```python
from build123d import *

# Parameters (mm, degrees)
SKETCH_1_W          = 70
SKETCH_1_H          = 40
EXTRUDE_1_DEPTH     = 5
CUT_EXTRUDE_1_DEPTH = 5
FILLET_1_R          = 2
SKETCH_3_W          = 23.333333333
SKETCH_3_H          = 4.8
EXTRUDE_2_DEPTH     = 5
FILLET_2_R          = 1
SKETCH_4_R          = 1.1
CUT_EXTRUDE_2_DEPTH = 5
HOLE_WIZARD_M3_1_D  = 3.4


with BuildPart() as part:
    # 草图1 → 凸台-拉伸1 (new body)
    with BuildSketch(Plane(origin=(0, 0, 0), x_dir=(0, 0, -1), z_dir=(1, 0, 0))):
        with Locations((35, 20)):
            Rectangle(SKETCH_1_W, SKETCH_1_H)
    extrude(amount=EXTRUDE_1_DEPTH)

    # 草图2 → 切除-拉伸1 (cut)
    with BuildSketch(Plane(origin=(5, 0, 0), x_dir=(0, 0, -1), z_dir=(1, 0, 0))):
        Polygon((8, 8), (24, 8), (8, 32), align=None)
        Polygon((31, 32), (31, 8), (15, 32), align=None)
        Polygon((39, 32), (39, 8), (55, 32), align=None)
        Polygon((62, 8), (62, 32), (46, 8), align=None)
    extrude(amount=-CUT_EXTRUDE_1_DEPTH, mode=Mode.SUBTRACT)

    # 圆角1
    fillet_1_edges = [part.edges().sort_by_distance(p)[0] for p in [
        (2.5, 32, -31),
        (2.5, 8, -31),
        (2.5, 32, -15),
        (2.5, 8, -39),
        (2.5, 32, -39),
        (2.5, 32, -55),
        (2.5, 32, -62),
        (2.5, 8, -62),
        (2.5, 8, -46),
        (2.5, 8, -8),
        (2.5, 32, -8),
        (2.5, 8, -24),
    ]]
    fillet(fillet_1_edges, radius=FILLET_1_R)

    # 草图3 → 凸台-拉伸2 (add)
    with BuildSketch(Plane(origin=(5, 0, 0), x_dir=(0, 0, -1), z_dir=(1, 0, 0))):
        with Locations((11.666666667, 42.4)):
            Rectangle(SKETCH_3_W, SKETCH_3_H)
        with Locations((58.333333334, 42.4)):
            Rectangle(SKETCH_3_W, SKETCH_3_H)
        with Locations((58.333333334, -2.4)):
            Rectangle(SKETCH_3_W, SKETCH_3_H)
        with Locations((11.666666667, -2.4)):
            Rectangle(SKETCH_3_W, SKETCH_3_H)
    extrude(amount=-EXTRUDE_2_DEPTH)

    # 圆角2
    fillet_2_edges = [part.edges().sort_by_distance(p)[0] for p in [
        (2.5, 44.8, 0),
        (2.5, 44.8, -23.333333333),
        (2.5, 44.8, -70),
        (2.5, 44.8, -46.666666667),
        (2.5, -4.8, -23.333333333),
        (2.5, -4.8, 0),
        (2.5, -4.8, -70),
        (2.5, -4.8, -46.666666667),
    ]]
    fillet(fillet_2_edges, radius=FILLET_2_R)

    # 草图4 → 切除-拉伸2 (cut)
    with BuildSketch(Plane(origin=(5, 0, 0), x_dir=(0, 0, -1), z_dir=(1, 0, 0))):
        with Locations((23.333333333, 40)):
            Circle(SKETCH_4_R)
        with Locations((46.666666667, 40)):
            Circle(SKETCH_4_R)
        with Locations((46.666666667, 0)):
            Circle(SKETCH_4_R)
        with Locations((23.333333333, 0)):
            Circle(SKETCH_4_R)
    extrude(amount=-CUT_EXTRUDE_2_DEPTH, mode=Mode.SUBTRACT)

    # M3 间隙孔1 (through all)
    with Locations(Plane(origin=(5, 0, 0), x_dir=(0, 0, -1), z_dir=(1, 0, 0))):
        with Locations((57.5, 37), (47.5, 37), (57.5, 3), (47.5, 3), (22.5, 3), (12.5, 3), (22.5, 37), (12.5, 37)):
            Hole(HOLE_WIZARD_M3_1_D / 2)


solid = part.part
```
Here's how the part is built. I have some questions about the finished solid (model axes, mm). Coordinates: 2 decimals unless noted, no trailing zeros. Order: outer loops, then holes, each group sorted by start corner. A loop starts at its lowest first (then second) coordinate and runs counter-clockwise, first axis right, second up. Notation, with made-up numbers: (24.5, -37.5) -> (73.5, -37.5) arc R35 cw to (73.5, -4.5) -> close; hole circle Ø5 at (62.25, -24.75). An arc over 180 degrees is marked (long way). Return JSON: item names as keys, results as strings.
1) If we section it at B-B on z = -15: List the corners of the cut face in (x, y) for me.
Conclusion:
{"outline": "(0, -4.8) -> (5, -4.8) -> (5, 8) -> (0, 8) -> close; (0, 21.5) -> (5, 21.5) -> (5, 44.8) -> (0, 44.8) -> close"}
2) If we section it at D-D on x = 3.6: State how many separate pieces and enclosed holes the cut face has, plus the area to 3 significant figures.
Conclusion:
{"separate pieces": "1", "enclosed holes": "12", "area": "2,440 mm²"}
3) If we section it at A-A on y = 37: List the corners of the cut face in (x, z) for me, plus the area to 3 significant figures.
Conclusion:
{"outline": "(0, -70) -> (5, -70) -> (5, -59.2) -> (0, -59.2) -> close; (0, -55.8) -> (5, -55.8) -> (5, -49.2) -> (0, -49.2) -> close; (0, -45.8) -> (5, -45.8) -> (5, -24.2) -> (0, -24.2) -> close; (0, -20.8) -> (5, -20.8) -> (5, -14.2) -> (0, -14.2) -> close; (0, -10.8) -> (5, -10.8) -> (5, 0) -> (0, 0) -> close", "area": "282 mm²"}
4) Thinking about a two-plate mould opening in Y: for faces 1 (the flat face through (3, 20, 0)), 2 (the cylindrical face through (2.47, 3.07, -59.2)), 3 (the cylindrical face through (2.54, 0.8, -22.58)), 4 (the flat face through (3, 44.8, -12)), which applies, +Y half, -Y half, draft (parallel to the pull), parting line (faces both ways), or undercut?
Conclusion:
{"face 1": "draft", "face 2": "undercut", "face 3": "undercut", "face 4": "+Y half"}
5) If I drill on probe 1 along Y at (x, z) = (4.55, -29); probe 2 along Y at (x, z) = (4.1, -48); probe 3 along Z at (x, y) = (0.35, 27.5), over which ranges is the centre line in solid material (lowest first)?
Conclusion:
{"probe 1": "y = 0 to 12.61, 32 to 40", "probe 2": "y = -4.8 to 1.38, 4.62 to 9.01, 10.99 to 21.5, 32 to 35.38, 38.62 to 44.8", "probe 3": "z = -70 to -52, -39 to -31, -18 to 0"}
6) If we section it at C-C on z = -57.5: List the corners of the cut face in (x, y) for me, plus the area to 3 significant figures.
Conclusion:
{"outline": "(0, -4.8) -> (5, -4.8) -> (5, 1.3) -> (0, 1.3) -> close; (0, 4.7) -> (5, 4.7) -> (5, 8) -> (0, 8) -> close; (0, 25.25) -> (5, 25.25) -> (5, 35.3) -> (0, 35.3) -> close; (0, 38.7) -> (5, 38.7) -> (5, 44.8) -> (0, 44.8) -> close", "area": "128 mm²"}
7) I'm going to push flat-ended pins straight in: P1, Ø12, axis at y = 28, z = -54.5, coming from the -X side; P2, Ø1.5, axis at x = 3.5, z = -26, coming from the -Y side. Where does each tip first touch, or does it pass through?
Conclusion:
{"P1": "stops at x = 0", "P2": "stops at y = 0"}
